```python
from build123d import *

# Parameters (mm, degrees)
SKETCH1_R               = 2.6035
BOSS_EXTRUDE1_DEPTH     = 457.2
CUT_EXTRUDE2_DEPTH      = 4.318
CUT_EXTRUDE2_DEPTH_BACK = 26.924
SKETCH5_W               = 400.863196081
SKETCH5_H               = 43.327238712
CUT_EXTRUDE3_DEPTH      = 26.4


with BuildPart() as part:
    # Sketch1 → Boss-Extrude1 (new body, symmetric)
    with BuildSketch(Plane.XY):
        with BuildLine():
            Line((-7.179650497, -8.645192506), (-3.952270251, -5.423690499))
            ThreePointArc((-3.952270251, -5.423690499), (-2.922936451, -4.736929036), (-1.709253557, -4.4958))
            Line((-1.709253557, -4.4958), (1.709253557, -4.4958))
            ThreePointArc((1.709253557, -4.4958), (2.922936451, -4.736929036), (3.952270251, -5.423690499))
            Line((3.952270251, -5.423690499), (7.179650497, -8.645192506))
            ThreePointArc((7.179650497, -8.645192506), (7.41473083, -9.822813117), (6.416408329, -10.4902))
            Line((6.416408329, -10.4902), (4.287512407, -10.4902))
            ThreePointArc((4.287512407, -10.4902), (3.54574862, -10.79744862), (3.2385, -11.539212407))
            Line((3.2385, -11.539212407), (3.2385, -11.650987593))
            ThreePointArc((3.2385, -11.650987593), (3.54574862, -12.39275138), (4.287512407, -12.7))
            Line((4.287512407, -12.7), (5.317126718, -12.7))
            ThreePointArc((5.317126718, -12.7), (5.825126718, -12.192), (6.333126718, -12.7))
            Line((6.333126718, -12.7), (9.550443118, -12.7))
            ThreePointArc((9.550443118, -12.7), (10.058366869, -12.192000006), (10.566443095, -12.699847501))
            ThreePointArc((10.566443095, -12.699847501), (12.082537762, -12.08250727), (12.699846982, -10.566399977))
            ThreePointArc((12.699846982, -10.566399977), (12.192000006, -10.058323491), (12.7, -9.5504))
            Line((12.7, -9.5504), (12.7, -6.3330836))
            ThreePointArc((12.7, -6.3330836), (12.192, -5.8250836), (12.7, -5.3170836))
            Line((12.7, -5.3170836), (12.7, -4.287469289))
            ThreePointArc((12.7, -4.287469289), (12.39275138, -3.545705502), (11.650987593, -3.238456882))
            Line((11.650987593, -3.238456882), (11.539212407, -3.238456882))
            ThreePointArc((11.539212407, -3.238456882), (10.79744862, -3.545705502), (10.4902, -4.287469289))
            Line((10.4902, -4.287469289), (10.4902, -6.402089023))
            ThreePointArc((10.4902, -6.402089023), (9.856505071, -7.351067942), (8.737131347, -7.129408934))
            Line((8.737131347, -7.129408934), (5.441005833, -3.840816462))
            ThreePointArc((5.441005833, -3.840816462), (4.750877967, -2.809883091), (4.5085, -1.593185507))
            Line((4.5085, -1.593185507), (4.5085, 1.593185507))
            ThreePointArc((4.5085, 1.593185507), (4.750877967, 2.809883091), (5.441005833, 3.840816462))
            Line((5.441005833, 3.840816462), (8.737131347, 7.129408934))
            ThreePointArc((8.737131347, 7.129408934), (9.856505071, 7.351067942), (10.4902, 6.402089023))
            Line((10.4902, 6.402089023), (10.4902, 4.287469289))
            ThreePointArc((10.4902, 4.287469289), (10.79744862, 3.545705502), (11.539212407, 3.238456882))
            Line((11.539212407, 3.238456882), (11.650987593, 3.238456882))
            ThreePointArc((11.650987593, 3.238456882), (12.39275138, 3.545705502), (12.7, 4.287469289))
            Line((12.7, 4.287469289), (12.7, 5.3170836))
            ThreePointArc((12.7, 5.3170836), (12.192, 5.8250836), (12.7, 6.3330836))
            Line((12.7, 6.3330836), (12.7, 9.5504))
            ThreePointArc((12.7, 9.5504), (12.192000006, 10.058323491), (12.699846982, 10.566399977))
            ThreePointArc((12.699846982, 10.566399977), (12.082537762, 12.08250727), (10.566443095, 12.699847501))
            ThreePointArc((10.566443095, 12.699847501), (10.058366869, 12.192000006), (9.550443118, 12.7))
            Line((9.550443118, 12.7), (6.333126718, 12.7))
            ThreePointArc((6.333126718, 12.7), (5.825126718, 12.192), (5.317126718, 12.7))
            Line((5.317126718, 12.7), (4.287512407, 12.7))
            ThreePointArc((4.287512407, 12.7), (3.54574862, 12.39275138), (3.2385, 11.650987593))
            Line((3.2385, 11.650987593), (3.2385, 11.539212407))
            ThreePointArc((3.2385, 11.539212407), (3.54574862, 10.79744862), (4.287512407, 10.4902))
            Line((4.287512407, 10.4902), (6.476788598, 10.4902))
            ThreePointArc((6.476788598, 10.4902), (7.432222385, 9.85140422), (7.207036008, 8.724370562))
            Line((7.207036008, 8.724370562), (3.898272566, 5.423169045))
            ThreePointArc((3.898272566, 5.423169045), (2.869120213, 4.736787962), (1.655778399, 4.4958))
            Line((1.655778399, 4.4958), (-1.655778399, 4.4958))
            ThreePointArc((-1.655778399, 4.4958), (-2.869120213, 4.736787962), (-3.898272566, 5.423169045))
            Line((-3.898272566, 5.423169045), (-7.207036008, 8.724370562))
            ThreePointArc((-7.207036008, 8.724370562), (-7.432222385, 9.85140422), (-6.476788598, 10.4902))
            Line((-6.476788598, 10.4902), (-4.287512407, 10.4902))
            ThreePointArc((-4.287512407, 10.4902), (-3.54574862, 10.79744862), (-3.2385, 11.539212407))
            Line((-3.2385, 11.539212407), (-3.2385, 11.650987593))
            ThreePointArc((-3.2385, 11.650987593), (-3.54574862, 12.39275138), (-4.287512407, 12.7))
            Line((-4.287512407, 12.7), (-5.317126718, 12.7))
            ThreePointArc((-5.317126718, 12.7), (-5.825126718, 12.192), (-6.333126718, 12.7))
            Line((-6.333126718, 12.7), (-9.550443118, 12.7))
            ThreePointArc((-9.550443118, 12.7), (-10.058366869, 12.192000006), (-10.566443095, 12.699847501))
            ThreePointArc((-10.566443095, 12.699847501), (-12.082537762, 12.08250727), (-12.699846982, 10.566399977))
            ThreePointArc((-12.699846982, 10.566399977), (-12.192000006, 10.058323491), (-12.7, 9.5504))
            Line((-12.7, 9.5504), (-12.7, 6.3330836))
            ThreePointArc((-12.7, 6.3330836), (-12.192, 5.8250836), (-12.7, 5.3170836))
            Line((-12.7, 5.3170836), (-12.7, 4.287469289))
            ThreePointArc((-12.7, 4.287469289), (-12.39275138, 3.545705502), (-11.650987593, 3.238456882))
            Line((-11.650987593, 3.238456882), (-11.539212407, 3.238456882))
            ThreePointArc((-11.539212407, 3.238456882), (-10.79744862, 3.545705502), (-10.4902, 4.287469289))
            Line((-10.4902, 4.287469289), (-10.4902, 6.402089023))
            ThreePointArc((-10.4902, 6.402089023), (-9.856505071, 7.351067942), (-8.737131347, 7.129408934))
            Line((-8.737131347, 7.129408934), (-5.441005833, 3.840816462))
            ThreePointArc((-5.441005833, 3.840816462), (-4.750877967, 2.809883091), (-4.5085, 1.593185507))
            Line((-4.5085, 1.593185507), (-4.5085, -1.593185507))
            ThreePointArc((-4.5085, -1.593185507), (-4.750877967, -2.809883091), (-5.441005833, -3.840816462))
            Line((-5.441005833, -3.840816462), (-8.737131347, -7.129408934))
            ThreePointArc((-8.737131347, -7.129408934), (-9.856505071, -7.351067942), (-10.4902, -6.402089023))
            Line((-10.4902, -6.402089023), (-10.4902, -4.287469289))
            ThreePointArc((-10.4902, -4.287469289), (-10.79744862, -3.545705502), (-11.539212407, -3.238456882))
            Line((-11.539212407, -3.238456882), (-11.650987593, -3.238456882))
            ThreePointArc((-11.650987593, -3.238456882), (-12.39275138, -3.545705502), (-12.7, -4.287469289))
            Line((-12.7, -4.287469289), (-12.7, -5.3170836))
            ThreePointArc((-12.7, -5.3170836), (-12.192, -5.8250836), (-12.7, -6.3330836))
            Line((-12.7, -6.3330836), (-12.7, -9.5504))
            ThreePointArc((-12.7, -9.5504), (-12.192000006, -10.058323491), (-12.699846982, -10.566399977))
            ThreePointArc((-12.699846982, -10.566399977), (-12.082537762, -12.08250727), (-10.566443095, -12.699847501))
            ThreePointArc((-10.566443095, -12.699847501), (-10.058366869, -12.192000006), (-9.550443118, -12.7))
            Line((-9.550443118, -12.7), (-6.333126718, -12.7))
            ThreePointArc((-6.333126718, -12.7), (-5.825126718, -12.192), (-5.317126718, -12.7))
            Line((-5.317126718, -12.7), (-4.287512407, -12.7))
            ThreePointArc((-4.287512407, -12.7), (-3.54574862, -12.39275138), (-3.2385, -11.650987593))
            Line((-3.2385, -11.650987593), (-3.2385, -11.539212407))
            ThreePointArc((-3.2385, -11.539212407), (-3.54574862, -10.79744862), (-4.287512407, -10.4902))
            Line((-4.287512407, -10.4902), (-6.416408329, -10.4902))
            ThreePointArc((-6.416408329, -10.4902), (-7.41473083, -9.822813117), (-7.179650497, -8.645192506))
        make_face()
        Circle(SKETCH1_R, mode=Mode.SUBTRACT)
    extrude(amount=BOSS_EXTRUDE1_DEPTH, both=True)

    # Sketch3 → Cut-Extrude2 (cut, two sides)
    with BuildSketch(Plane.ZY.offset(12.7)) as cut_extrude2_sk:
        Polygon((-203.2, -27.552777595), (-203.2, 21.158109763), (-461.090893327, 21.158109763), (-461.090893327, -25.4), align=None)
    extrude(amount=CUT_EXTRUDE2_DEPTH, mode=Mode.SUBTRACT)
    extrude(cut_extrude2_sk.sketch, amount=-CUT_EXTRUDE2_DEPTH_BACK, mode=Mode.SUBTRACT)

    # Sketch5 → Cut-Extrude3 (cut, through all)
    with BuildSketch(Plane(origin=(12.7, 0, 0), x_dir=(0, 0, -1), z_dir=(1, 0, 0))):
        with Locations((7.887376468, 2.312510515)):
            Rectangle(SKETCH5_W, SKETCH5_H)
    extrude(amount=-CUT_EXTRUDE3_DEPTH, mode=Mode.SUBTRACT)


solid = part.part
```
Geometry: final body of the model. Coordinates: model frame, mm. Give positions to 0.01 mm unless a question says otherwise; leave off trailing zeros. Return JSON: item names as keys, results as strings.
Item 1: Line query: line 1 (Y direction, x = 0, z = 257.5); line 2 (X direction, y = 0, z = 365); line 3 (X direction, y = 5.5, z = 309). Output: solid intervals per line, ascending.
Filled in:
{"line 1": "-4.5 to -2.6, 2.6 to 4.5", "line 2": "-4.51 to -2.6, 2.6 to 4.51", "line 3": "-12.31 to -10.49, -7.1 to -3.98, 3.98 to 7.1, 10.49 to 12.31"}
Item 2: Mould query, pull axis Y, two halves, no side actions, for faces 1 (the flat face through (0, 3, 192.544)), 2 (the cylindrical face through (2.483, 0.782, 323.02)). Classes: released by +Y, released by -Y, zero draft, split by the parting line, or undercut.
Filled in:
{"face 1": "zero draft", "face 2": "undercut"}
Item 3: Pin query (flat end, axial travel): P1, Ø2, axis at x = 2, z = 270, coming from the +Y side; P2, Ø6, axis at x = -0.5, z = 287.5, coming from the +Y side; P3, Ø1.7, axis at x = -0.5, z = 332.5, coming from the -Y side; P4, Ø2, axis at x = 5, y = -8.5, coming from the +Z side. Return the tip coordinate at first contact, or that it passes through.
Filled in:
{"P1": "y = 4.79", "P2": "y = 12.34", "P3": "y = -4.5", "P4": "through"}
